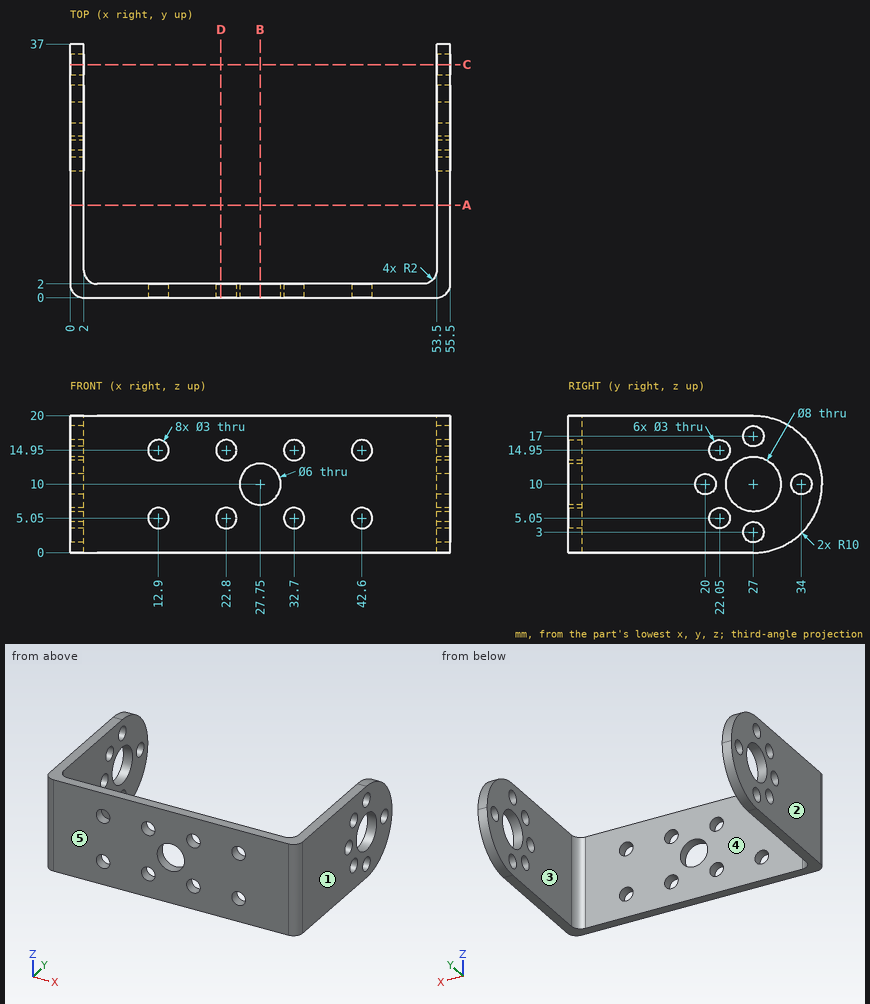
Job drawing, mm, ordinate dimensions from the low corner. One solid piece. A direction names the side the tool comes from. Coordinates: 2 decimals unless noted, no trailing zeros. Order: outer loops, then holes, each group sorted by start corner. A loop starts at its lowest first (then second) coordinate and runs counter-clockwise, first axis right, second up. Notation, with made-up numbers: M 86.5,85 L 124.5,85 A19 cw 124.5,122 Z; hole C 20.5,81.25 d4. An arc over 180 degrees is marked long. Return JSON: item names as keys, results as strings.
1. Flat gauge pins, fed straight in: pin 1 (1 mm diameter, centred on x = 45, z = 11, fed in from +Y); pin 2 (2.5 mm diameter, centred on y = 22.05, z = 14.95, fed in from -X). Where does each tip first touch, or does it go through?
Ans:
{"pin 1": "y = 2", "pin 2": "through"}
2. Saw through at C-C (y = 34). Give the cut face in (x, z).
Ans:
{"outline": "M 0,2.86 L 2,2.86 L 2,8.5 L 0,8.5 Z; M 0,11.5 L 2,11.5 L 2,17.14 L 0,17.14 Z; M 53.5,2.86 L 55.5,2.86 L 55.5,8.5 L 53.5,8.5 Z; M 53.5,11.5 L 55.5,11.5 L 55.5,17.14 L 53.5,17.14 Z"}
3. Saw through at D-D (x = 22). Give the cut face in (y, z).
Ans:
{"outline": "M 0,0 L 2,0 L 2,3.78 L 0,3.78 Z; M 0,6.32 L 2,6.32 L 2,13.68 L 0,13.68 Z; M 0,16.22 L 2,16.22 L 2,20 L 0,20 Z"}
4. Drill centre lines: probe 1 along X at (y, z) = (15, 8); probe 2 along Y at (x, z) = (26.5, 18.25); probe 3 along Z at (x, y) = (54, 34). Where is each one in solid material? Low to high.
Ans:
{"probe 1": "0 to 2, 53.5 to 55.5", "probe 2": "0 to 2", "probe 3": "2.86 to 8.5, 11.5 to 17.14"}
5. Saw through at B-B (x = 27.75). Give the cut face in (y, z), and give its area (3 significant figures).
Ans:
{"outline": "M 0,0 L 2,0 L 2,7 L 0,7 Z; M 0,13 L 2,13 L 2,20 L 0,20 Z", "area": "28.0 mm^2"}
6. Saw through at A-A (y = 13.5). Give the cut face in (x, z), and give its area (3 significant figures).
Ans:
{"outline": "M 0,0 L 2,0 L 2,20 L 0,20 Z; M 53.5,0 L 55.5,0 L 55.5,20 L 53.5,20 Z", "area": "80.0 mm^2"}
7. Tool access for the marked faces 4 and 5: list every direction of +Z, -Z, +X, -X, +Y, -Y with a clear straight run to the whole face (end or side of a thin tool).
Ans:
{"face 4": "+Z, -Z, +Y", "face 5": "+Z, -Z, +X, -X, -Y"}
8. Pull direction X, two halves, no side cores. Call the marked faces 1, 2 and 3: +X half, -X half, draft (parallel to the pull), parting line (faces both ways), or undercut.
Ans:
{"face 1": "+X half", "face 2": "-X half", "face 3": "undercut"}
